Could you check a few things on this model? Use its own coordinates, in mm. Round coordinates to 2 decimals unless told otherwise and drop trailing zeros. Put each result on its own line as item: value. Start each with the question number.
1. Imagine slicing it at A-A, the plane y = -0.45. Count the separate pieces of the cut face and the enclosed holes in it, and give its area (3 significant figures).
2. If we mould it in two halves opening along Z, with no side actions, what happens to faces 1 (the flat face through (0, -0.72, 0)), 2 (the flat face through (0, 0.7, 0))? For each: pulls with the +Z half, pulls with the -Z half, needs draft (parallel to the pull), parting line crosses it, or undercut.
3. I need wall thicknesses on line 1 (Z direction, x = 0.6, y = -0.15); line 2 (Y direction, x = 2.1, z = 1.5); line 3 (Z direction, x = -0.1, y = -0.2). Which ranges of each line are inside material? Lowest first, please. Write a range as [from, to].
4. I'm going to push flat-ended pins straight in: P1, Ø0.5, axis at y = 0, z = -2.5, coming from the +X side (3 decimals); P2, Ø0.5, axis at y = -0.5, z = 2.5, coming from the -X side (3 decimals). Where does each tip first touch, or does it pass through?
```python
from build123d import *

# Parameters (mm, degrees)
SKETCH1_W                = 5.5
SKETCH1_H                = 4.4
EXTRUDE1_DEPTH           = 0.7
EXTRUDE1_TAPER           = 12
EXTRUDE1_OTHER_WAY_DEPTH = 0.23
SKETCH2_W                = 5.5
SKETCH2_H                = 4.4
EXTRUDE2_DEPTH           = 0.49
EXTRUDE2_TAPER           = 12
CHAMFER1_SIZE            = 0.29360287
CHAMFER1_SIZE_2          = 0.3
SKETCH3_R                = 0.317461986
CUT_EXTRUDE1_DEPTH       = 0.15
CUT_EXTRUDE1_DRAFT       = -12
EXTRUDE3_START           = 0.635
EXTRUDE3_DEPTH           = 0.21
LPATTERN3_COUNT          = 2
LPATTERN3_PITCH          = 1.27
LPATTERN3_COL_COUNT      = 3
LPATTERN3_COL_PITCH      = 1.27
FILLET1_R                = 0.1
FILLET2_R                = 0.25


with BuildPart() as part:
    # Sketch1 → Extrude1 (new body)
    with BuildSketch(Plane(origin=(0, 0, 0), x_dir=(1, 0, 0), z_dir=(0, 1, 0))):
        Rectangle(SKETCH1_W, SKETCH1_H)
    extrude(amount=EXTRUDE1_DEPTH, taper=EXTRUDE1_TAPER)

    # Sketch1 → Extrude1 other way (add)
    with BuildSketch(Plane(origin=(0, 0, 0), x_dir=(1, 0, 0), z_dir=(0, 1, 0))):
        Rectangle(SKETCH1_W, SKETCH1_H)
    extrude(amount=-EXTRUDE1_OTHER_WAY_DEPTH)

    # Sketch2 → Extrude2 (add)
    with BuildSketch(Plane.XZ.offset(0.23)):
        Rectangle(SKETCH2_W, SKETCH2_H)
    extrude(amount=EXTRUDE2_DEPTH, taper=EXTRUDE2_TAPER)

    # Chamfer1
    # the kernel refuses this chamfer: 0.3, 0.29360287 mm, written as the material it takes off along each edge
    with BuildSketch(Plane(origin=(3.374914076, 0.7, -2.051210407), x_dir=(0, 0.025194664498195945, 0.9996825640576229), z_dir=(-1, 0, 0))) as chamfer1_piece_1:
        Polygon((CHAMFER1_SIZE * 0.999682563914, -CHAMFER1_SIZE * 0.0251946644946), (-CHAMFER1_SIZE_2 * 0.232489792804, -CHAMFER1_SIZE_2 * 0.972598836233), (0, 0), align=None)
    extrude(amount=6.749828151, mode=Mode.SUBTRACT)


with BuildPart() as cut_extrude1_tool:
    # Sketch3 → Cut-Extrude1 (with draft: the straight prism first)
    with BuildSketch(Plane(origin=(0, 0.7, 0), x_dir=(-1, 0, 0), z_dir=(0, 1, 0))):
        with Locations((-1.845269249, -0.967381419)):
            Circle(SKETCH3_R)
    extrude(amount=-CUT_EXTRUDE1_DEPTH)
    # Cut-Extrude1: the draft: its side faces are tilted about the plane it starts from
    cut_extrude1_sides = [cut_extrude1_tool.faces().sort_by_distance(p)[0] for p in [
        (2.162731235, 0.625, -0.967381419),
    ]]
    draft(cut_extrude1_sides, Plane(origin=(0, 0.7, 0), x_dir=(-1, 0, 0), z_dir=(0, 1, 0)), CUT_EXTRUDE1_DRAFT)


with BuildPart() as part_1:
    add(part.part)

    # Cut-Extrude1: cut by cut_extrude1_tool
    add(cut_extrude1_tool.part, mode=Mode.SUBTRACT)

    # Sketch4 → Extrude3 (add, symmetric)
    with BuildSketch(Plane(origin=(0, 0, 0), x_dir=(0, 0, -1), z_dir=(1, 0, 0)).offset(EXTRUDE3_START)):
        Polygon((-2.687449676, -0.75), (-2.608709879, 0.15), (2.608709879, 0.15), (2.687449676, -0.75), (3.15, -0.75), (3.15, -0.9), (2.55, -0.9), (2.471260203, 0), (-2.471260203, 0), (-2.55, -0.9), (-3.15, -0.9), (-3.15, -0.75), align=None)
    extrude3 = extrude(amount=EXTRUDE3_DEPTH, both=True)

    # LPattern3: Extrude3 ×2
    with Locations(*[(i * LPATTERN3_PITCH, 0, 0) for i in range(1, LPATTERN3_COUNT)]):
        add(extrude3)

    # LPattern3 col: Extrude3 ×3
    with Locations(*[(-i * LPATTERN3_COL_PITCH, 0, 0) for i in range(1, LPATTERN3_COL_COUNT)]):
        add(extrude3)

    # Fillet1
    fillet1_edges = [part_1.edges().sort_by_distance(p)[0] for p in [
        (-0.635, -0.75, 2.687449676),
        (-0.635, 0, 2.471260203),
        (-0.635, 0, -2.471260203),
        (-1.905, -0.75, -2.687449676),
        (-1.905, -0.75, 2.687449676),
        (-1.905, 0, 2.471260203),
        (-1.905, 0, -2.471260203),
        (1.905, -0.75, -2.687449676),
        (1.905, -0.75, 2.687449676),
        (1.905, 0, 2.471260203),
        (1.905, 0, -2.471260203),
        (0.635, -0.75, -2.687449676),
        (0.635, -0.75, 2.687449676),
        (0.635, 0, 2.471260203),
        (0.635, 0, -2.471260203),
        (-0.635, -0.75, -2.687449676),
    ]]
    fillet(fillet1_edges, radius=FILLET1_R)

    # Fillet2
    fillet2_edges = [part_1.edges().sort_by_distance(p)[0] for p in [
        (-0.635, -0.9, 2.55),
        (-0.635, -0.9, -2.55),
        (-1.905, 0.15, -2.608709879),
        (-1.905, 0.15, 2.608709879),
        (-1.905, -0.9, 2.55),
        (-1.905, -0.9, -2.55),
        (1.905, 0.15, -2.608709879),
        (1.905, 0.15, 2.608709879),
        (1.905, -0.9, 2.55),
        (1.905, -0.9, -2.55),
        (0.635, 0.15, -2.608709879),
        (0.635, 0.15, 2.608709879),
        (0.635, -0.9, -2.55),
        (-0.635, 0.15, -2.608709879),
        (-0.635, 0.15, 2.608709879),
    ]]
    fillet(fillet2_edges, radius=FILLET2_R)


solid = part_1.part
```
Entries:
1. separate pieces: 9
1. enclosed holes: 0
1. area: 23.8 mm^2
2. face 1: undercut
2. face 2: needs draft
3. line 1: [-2.63, -2.48], [-2.2, 2.2], [2.48, 2.63]
3. line 2: [-0.72, 0.7]
3. line 3: [-2.2, 2.2]
4. P1: x = 2.115
4. P2: x = -2.115
